Input: part model. Units: mm. Frame: model coordinates. Face numbers are marked on the shaded views. A direction names the side the tool comes from. Give positions to 0.01 mm unless a question says otherwise; leave off trailing zeros. Write each loop counter-clockwise with the first axis right and the second up, starting at its lowest first coordinate (ties: lowest second). Pieces come first, ordered by that corner, then holes. Notation, with made-up numbers: (2, -35.5) - (33, -35.5) arc R24 ccw to (33, 0.5) - close; hole circle Ø6 at (67, 70). An arc over 180 degrees is marked (long way). Use a Markdown table: item, result. Add a question column.
1. Set-up query: the marked faces 4, 5 and 6. Return all of +Z, -Z, +X, -X, +Y, -Y with unobstructed straight access to the full face (end or side cutting, diameter ignored); none if empty.
2. Section query A-A, the plane z = 2.5. Return loops of the section in (x, y) (3 decimals).
3. Section query B-B, the plane y = 7.5. Count the separate pieces of the cut face and the enclosed holes in it, plus the area to 3 significant figures.
4. Mould query, pull axis X, two halves, no side actions, for the marked faces 1, 2 and 3. Classes: released by +X, released by -X, zero draft, split by the parting line, or undercut.
5. Material intervals for probe 1 along Y at (x, z) = (-1.5, 0.75); probe 2 along Y at (x, z) = (26, 1.5); probe 3 along Z at (x, y) = (-7, 18.25), sorted ascending.
6. Pin query (flat end, axial travel): pin 1 (5 mm diameter, centred on x = 38.5, z = 1, fed in from +Y); pin 2 (4 mm diameter, centred on x = -2, z = 0.5, fed in from -Y); pin 3 (1.6 mm diameter, centred on x = -11.5, z = 0.5, fed in from -Y). Return the tip coordinate at first contact, or that it passes through.
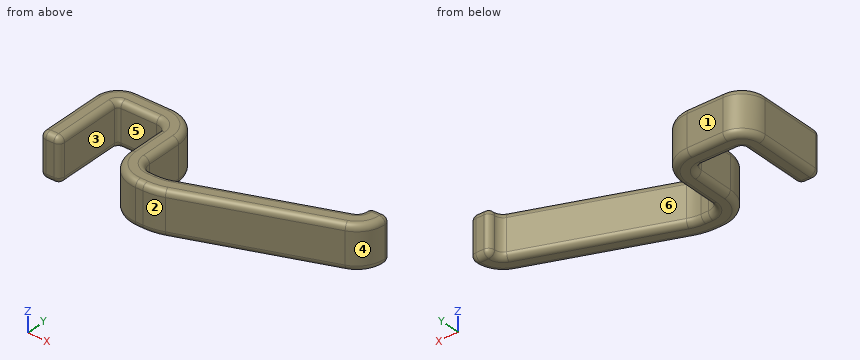
```python
from build123d import *

# Parameters (mm, degrees)
F1_W = 5
F1_H = 11
F3_R = 1.5


with BuildPart() as f2:
    # F2: sweep along a path in F0
    with BuildLine(Plane.XY) as f2_path:
        Line((-10.824024, 0), (-10.824024, 17))
        ThreePointArc((-10.824024, 17), (-9.945345, 19.12132), (-7.824024, 20))
        Line((-7.824024, 20), (1.175976, 20))
        ThreePointArc((1.175976, 20), (4.71151, 18.535534), (6.175976, 15))
        Line((6.175976, 15), (6.175976, 6))
        ThreePointArc((6.175976, 6), (7.933335, 1.757359), (12.175976, 0))
        Line((12.175976, 0), (13.999961, 0))
        ThreePointArc((13.999961, 0), (16.141058, 0.192557), (18.213442, 0.76405))
        Line((18.213442, 0.76405), (52.931593, 13.783356))
        ThreePointArc((52.931593, 13.783356), (55.285604, 15.617028), (56.175976, 18.465002))
        Line((56.175976, 18.465002), (56.175976, 20))
    # F1 (on Front) → F2 (sweep)
    with BuildSketch(Plane.XZ):
        with Locations((-11.190739, -0.00427)):
            Rectangle(F1_W, F1_H)
    sweep(path=f2_path.line)

    # F3
    f3_edges = [f2.edges().sort_by_distance(p)[0] for p in [
        (-8.690739, 8.5, 5.49573),
        (-11.190739, 0, 5.49573),
        (-13.690739, 8.5, 5.49573),
        (-11.972418, 21.148394, 5.49573),
        (-3.324024, 22.866714, 5.49573),
        (6.738583, 20.562607, 5.49573),
        (9.04269, 10.5, 5.49573),
        (9.960408, 3.784433, 5.49573),
        (13.087968, 2.866714, 5.49573),
        (15.629565, 3.013271, 5.49573),
        (34.565947, 9.957892, 5.49573),
        (52.929378, 17.249894, 5.49573),
        (53.309261, 19.232501, 5.49573),
        (55.809261, 20, 5.49573),
        (58.309261, 19.232501, 5.49573),
        (57.039006, 14.40192, 5.49573),
        (36.321564, 5.276246, 5.49573),
        (16.521689, -1.906496, 5.49573),
        (13.087968, -2.133286, 5.49573),
        (6.424874, 0.248899, 5.49573),
        (4.04269, 10.5, 5.49573),
        (3.203049, 17.027073, 5.49573),
        (-3.324024, 17.866714, 5.49573),
        (-8.436884, 17.61286, 5.49573),
        (-13.690739, 0, -0.00427),
        (-13.690739, 8.5, -5.50427),
        (-13.690739, 17, -0.00427),
        (-11.190739, 0, -5.50427),
        (-8.690739, 8.5, -5.50427),
        (-8.436884, 17.61286, -5.50427),
        (-3.324024, 17.866714, -5.50427),
        (3.203049, 17.027073, -5.50427),
        (4.04269, 10.5, -5.50427),
        (6.424874, 0.248899, -5.50427),
        (13.087968, -2.133286, -5.50427),
        (16.521689, -1.906496, -5.50427),
        (36.321564, 5.276246, -5.50427),
        (57.039006, 14.40192, -5.50427),
        (58.309261, 19.232501, -5.50427),
        (55.809261, 20, -5.50427),
        (53.309261, 19.232501, -5.50427),
        (52.929378, 17.249894, -5.50427),
        (34.565947, 9.957892, -5.50427),
        (15.629565, 3.013271, -5.50427),
        (13.087968, 2.866714, -5.50427),
        (9.960408, 3.784433, -5.50427),
        (9.04269, 10.5, -5.50427),
        (6.738583, 20.562607, -5.50427),
        (-3.324024, 22.866714, -5.50427),
        (-11.972418, 21.148394, -5.50427),
        (-8.690739, 0, -0.00427),
        (-8.690739, 17, -0.00427),
        (-7.824024, 22.866714, -0.00427),
        (-7.824024, 17.866714, -0.00427),
        (1.175976, 22.866714, -0.00427),
        (1.175976, 17.866714, -0.00427),
        (9.04269, 15, -0.00427),
        (4.04269, 15, -0.00427),
        (9.04269, 6, -0.00427),
        (4.04269, 6, -0.00427),
        (12.175976, 2.866714, -0.00427),
        (12.175976, -2.133286, -0.00427),
        (13.999961, 2.866714, -0.00427),
        (13.999961, -2.133286, -0.00427),
        (17.206871, 3.448238, -0.00427),
        (18.962489, -1.233408, -0.00427),
        (51.925022, 16.467545, -0.00427),
        (53.680639, 11.785899, -0.00427),
        (53.309261, 18.465002, -0.00427),
        (58.309261, 18.465002, -0.00427),
        (53.309261, 20, -0.00427),
        (58.309261, 20, -0.00427),
    ]]
    fillet(f3_edges, radius=F3_R)


solid = f2.part
```
Result sheet:
| question | item | result |
|---|---|---|
| 1 | face 4 | +Z, -Z, +X, -Y |
| 1 | face 5 | +Z, -Z, -Y |
| 1 | face 6 | +Z, -Z, +Y |
| 2 | outline | (-13.691, 1.5) arc R1.5 ccw to (-12.191, 0) - (-10.191, 0) arc R1.5 ccw to (-8.691, 1.5) - (-8.691, 17) arc R0.867 cw to (-7.824, 17.867) - (1.176, 17.867) arc R2.867 cw to (4.043, 15) - (4.043, 6) arc R8.133 ccw to (12.176, -2.133) - (14, -2.133) arc R14.133 ccw to (18.962, -1.233) - (53.681, 11.786) arc R7.133 ccw to (58.309, 18.465) - (58.309, 18.5) arc R1.5 ccw to (56.809, 20) - (54.809, 20) arc R1.5 ccw to (53.309, 18.5) - (53.309, 18.465) arc R2.133 cw to (51.925, 16.468) - (17.207, 3.448) arc R9.133 cw to (14, 2.867) - (12.176, 2.867) arc R3.133 cw to (9.043, 6) - (9.043, 15) arc R7.867 ccw to (1.176, 22.867) - (-7.824, 22.867) arc R5.867 ccw to (-13.691, 17) - close |
| 3 | separate pieces | 3 |
| 3 | enclosed holes | 0 |
| 3 | area | 257 mm² |
| 4 | face 1 | zero draft |
| 4 | face 2 | released by +X |
| 4 | face 3 | undercut |
| 5 | probe 1 | y = 17.87 to 22.87 |
| 5 | probe 2 | y = 1.41 to 6.75 |
| 5 | probe 3 | z = -5.01 to 5 |
| 6 | pin 1 | stops at y = 12.37 |
| 6 | pin 2 | stops at y = 17.87 |
| 6 | pin 3 | stops at y = 0 |
